Build history of the part. All positions in model axes, mm. Face numbers are marked on the shaded views. A direction names the side the tool comes from. Round coordinates to 2 decimals unless told otherwise and drop trailing zeros. Write each loop counter-clockwise with the first axis right and the second up, starting at its lowest first coordinate (ties: lowest second). Pieces come first, ordered by that corner, then holes. Notation, with made-up numbers: (13.5, -18.5) -> (71.5, -18.5) arc R22 cw to (71.5, -12.5) -> close; hole circle Ø7 at (-6.5, -0.5). An arc over 180 degrees is marked (long way). One line per question, with ' | ' between items.
from build123d import *

# Parameters (mm, degrees)
SKETCH1_W           = 28.3
SKETCH1_H           = 42
BOSS_EXTRUDE1_DEPTH = 4
SKETCH2_W           = 15
SKETCH2_H           = 15
CUT_EXTRUDE1_DEPTH  = 3
DRAFT1_ANGLE        = 30
FILLET1_R           = 2
SKETCH4_W           = 28.3
SKETCH4_H           = 42
SKETCH4_W_2         = 24.7
SKETCH4_H_2         = 38.4
BOSS_EXTRUDE2_DEPTH = 4
FILLET2_R           = 2.5


with BuildPart() as part:
    # Sketch1 → Boss-Extrude1 (new body)
    with BuildSketch(Plane(origin=(0, 0, 0), x_dir=(1, 0, 0), z_dir=(0, 1, 0))):
        with Locations((14.15, 21)):
            Rectangle(SKETCH1_W, SKETCH1_H)
    extrude(amount=BOSS_EXTRUDE1_DEPTH)

    # Sketch2 → Cut-Extrude1 (cut)
    with BuildSketch(Plane(origin=(0, 4, 0), x_dir=(1, 0, 0), z_dir=(0, 1, 0))):
        with Locations((14.15, 27.24)):
            Rectangle(SKETCH2_W, SKETCH2_H)
    extrude(amount=-CUT_EXTRUDE1_DEPTH, mode=Mode.SUBTRACT)

    # Draft1
    draft1_faces = [part.faces().sort_by_distance(p)[0] for p in [
        (6.65, 2.5, -27.24),
        (14.15, 2.5, -19.74),
        (21.65, 2.5, -27.24),
        (14.15, 2.5, -34.74),
    ]]
    draft(draft1_faces, Plane.ZX.offset(4), DRAFT1_ANGLE)

    # Fillet1
    fillet1_edges = [part.edges().sort_by_distance(p)[0] for p in [
        (8.382050808, 1, -27.24),
        (14.15, 1, -33.007949192),
        (19.917949192, 1, -27.24),
        (14.15, 1, -21.472050808),
    ]]
    fillet(fillet1_edges, radius=FILLET1_R)

    # Sketch4 → Boss-Extrude2 (add)
    with BuildSketch(Plane(origin=(0, 4, 0), x_dir=(1, 0, 0), z_dir=(0, 1, 0))):
        with Locations((14.15, 21)):
            Rectangle(SKETCH4_W, SKETCH4_H)
        with Locations((14.15, 21)):
            Rectangle(SKETCH4_W_2, SKETCH4_H_2, mode=Mode.SUBTRACT)
    extrude(amount=BOSS_EXTRUDE2_DEPTH)

    # Fillet2
    fillet2_edges = [part.edges().sort_by_distance(p)[0] for p in [
        (1.8, 4, -21),
        (26.5, 4, -21),
        (14.15, 4, -40.2),
        (26.5, 6, -40.2),
        (1.8, 6, -40.2),
    ]]
    fillet(fillet2_edges, radius=FILLET2_R)


solid = part.part
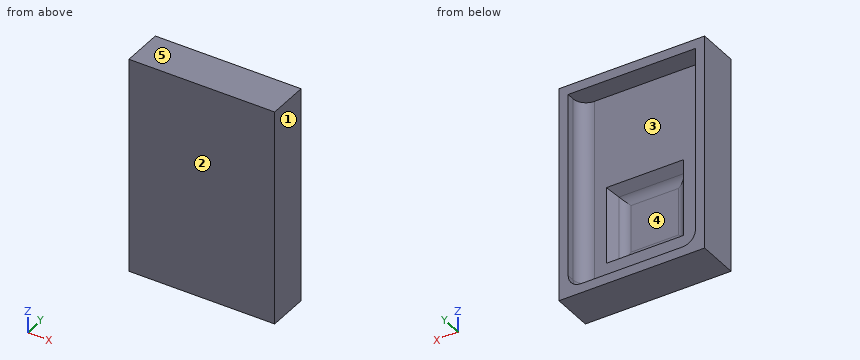
(1) Slice it at B-B (y = 3.5). Write the cut outline in (x, z).
Calculated:
outline: (0, -42) -> (28.3, -42) -> (28.3, 0) -> (0, 0) -> close; hole (6.94, -34.45) -> (21.36, -34.45) -> (21.36, -20.03) -> (6.94, -20.03) -> close
(2) Slice it at D-D (x = 22.25). Write the cut outline in (y, z).
Calculated:
outline: (0, -42) -> (8, -42) -> (8, -40.2) -> (6.5, -40.2) arc R2.5 cw to (4, -37.7) -> (4, -1.8) -> (8, -1.8) -> (8, 0) -> (0, 0) -> close
(3) Mould opens along X. For the marked faces 1, 2 and 3 say: pulls with the +X half, pulls with the -X half, needs draft (parallel to the pull), parting line crosses it, or undercut.
Calculated:
face 1: pulls with the +X half | face 2: needs draft | face 3: undercut
(4) Wall check: line 1 (X direction, y = 7.25, z = -28.5); line 2 (Y direction, x = 11, z = -29.5); line 3 (Y direction, x = 23, z = -32.5). Give the ranges that are in metal, low to high. Write a range as from..to.
Calculated:
line 1: 0..1.8, 26.5..28.3 | line 2: 0..1 | line 3: 0..4
(5) Drop flat-ended pins along their axis: pin 1 (3 mm diameter, centred on x = 5, z = -31, fed in from +Y); pin 2 (6 mm diameter, centred on x = 13.5, z = -20.5, fed in from +Y); pin 3 (3 mm diameter, centred on x = 15, z = -29, fed in from +Y). Give the stop position or say it passes through.
Calculated:
pin 1: y = 4.13 | pin 2: y = 4 | pin 3: y = 1
(6) 3-axis set-ups, long thin cutter, end or side, ignore diameter. For the marked faces 4 and 5: which of +Z, -Z, +X, -X, +Y, -Y reach the whole face in a straight line?
Calculated:
face 4: +Y | face 5: +Z, +X, -X, +Y, -Y
(7) Slice it at A-A (x = 15.25). Write the cut outline in (y, z), then the cut area to 3 significant figures.
Calculated:
outline: (0, -42) -> (8, -42) -> (8, -40.2) -> (6.5, -40.2) arc R2.5 cw to (4, -37.7) -> (4, -34.74) -> (2, -33.59) arc R2 cw to (1, -31.85) -> (1, -22.63) arc R2 cw to (2, -20.89) -> (4, -19.74) -> (4, -1.8) -> (8, -1.8) -> (8, 0) -> (0, 0) -> close | area: 144 mm2
(8) Slice it at C-C (z = -16). Write the cut outline in (x, y), then the cut area to 3 significant figures.
Calculated:
outline: (0, 0) -> (28.3, 0) -> (28.3, 8) -> (26.5, 8) -> (26.5, 6.5) arc R2.5 cw to (24, 4) -> (4.3, 4) arc R2.5 cw to (1.8, 6.5) -> (1.8, 8) -> (0, 8) -> close | area: 130 mm2
